Source: CAD feature listing. Evaluate the final solid. Frame: model axes, mm. Coordinates: 2 decimals unless noted, no trailing zeros. Write each loop counter-clockwise with the first axis right and the second up, starting at its lowest first coordinate (ties: lowest second). Pieces come first, ordered by that corner, then holes. Notation, with made-up numbers: M -7,-17 L -1,-17 A21 cw -1,20 Z; hole C 18.5,78.25 d6. An arc over 180 degrees is marked long. Write item = value, one per line. Start each with the question number.
1. Pin query (flat end, axial travel): pin 1 Ø5 at (x, y) = (0, 0) entering from -Z; pin 2 Ø2 at (x, z) = (3.5, 2) entering from -Y; pin 3 Ø1 at (x, z) = (-1, 3) entering from +Y; pin 4 Ø2 at (y, z) = (-3, 6.5) entering from -X. Return the tip coordinate at first contact, or that it passes through.
2. Section query A-A (y = 0). Output: boundary loops of the cut face in (x, z) (3 decimals), then the cut area to 3 significant figures.
3. Line query: line 1 along Y through (x, z) = (0, 6.25) (3 decimals); line 2 along Z through (x, y) = (0, 5); line 3 along Y through (x, z) = (0, 4.5) (3 decimals). Output: solid intervals per line, ascending.
4. Section query D-D (y = 7.75). Output: boundary loops of the cut face in (x, z).
5. Pull-direction query (Y, two-part tool) for faces 1 (the face through (0.34, -9.22, 3.88)), 2 (the face through (0.41, -3.15, 3.99)), 3 (the face through (-2.75, -12.4, 3.88)), 4 (the face through (0.662, 7.613, 2.297)); classes: pulls with the +Y half, pulls with the -Y half, needs draft (parallel to the pull), parting line crosses it, or undercut.
6. Section query B-B (x = 0). Output: boundary loops of the cut face in (y, z) (3 decimals).
```python
from build123d import *

# Parameters (mm, degrees)
SKETCH1_R                  = 12.7
BOSS_EXTRUDE1_DEPTH        = 7.874
F_1_4_0_2500_DOWEL_HOLE1_D = 6.35
F_1_8_0_1250_DOWEL_HOLE1_D = 3.175


with BuildPart() as part:
    # Sketch1 → Boss-Extrude1 (new body)
    with BuildSketch(Plane.XY):
        Circle(SKETCH1_R)
    extrude(amount=BOSS_EXTRUDE1_DEPTH)

    # 1/4 (0.2500) Dowel Hole1 (through all)
    with Locations(Plane(origin=(0, 0, 0), x_dir=(1, 0, 0), z_dir=(0, 0, -1))):
        with Locations((0, 0)):
            Hole(F_1_4_0_2500_DOWEL_HOLE1_D / 2)

    # 1/8 (0.1250) Dowel Hole1 (through all)
    with Locations(Plane.XY.offset(7.874)):
        with Locations((0, -7.669668031)):
            Hole(F_1_8_0_1250_DOWEL_HOLE1_D / 2)

    # Sketch7 → #8-32 Tapped Hole1 (revolve, cut)
    with BuildSketch(Plane(origin=(0, 0, 3.892930906), x_dir=(0, 0, -1), z_dir=(1, 0, 0))):
        Polygon((0, 0), (0, 13.97), (1.7272, 12.932193539), (1.7272, 0), align=None)
    revolve(axis=Axis((0, -6.35, 3.892930906), (0, 1, 0)), mode=Mode.SUBTRACT)


solid = part.part
```
Results are:
q1.pin_1 = through
q1.pin_2 = -12.45
q1.pin_3 = 12.66
q1.pin_4 = -12.54
q2.outline = M -12.7,0 L -3.175,0 L -3.175,7.874 L -12.7,7.874 Z; M 3.175,0 L 12.7,0 L 12.7,7.874 L 3.175,7.874 Z
q2.area = 150 mm^2
q3.line_1 = -12.7 to -9.257, -6.082 to -3.175, 3.175 to 12.7
q3.line_2 = 0 to 2.17, 5.62 to 7.87
q3.line_3 = -12.7 to -9.257, -6.082 to -3.175
q4.outline = M -10.06,0 L 10.06,0 L 10.06,7.87 L -10.06,7.87 Z; hole C 0,3.89 d3.45
q5.face_1 = undercut
q5.face_2 = undercut
q5.face_3 = parting line crosses it
q5.face_4 = needs draft
q6.outline = M -12.7,0 L -9.257,0 L -9.257,7.874 L -12.7,7.874 Z; M -6.082,0 L -3.175,0 L -3.175,7.874 L -6.082,7.874 Z; M 3.175,0 L 12.7,0 L 12.7,2.166 L 3.175,2.166 Z; M 3.175,5.62 L 12.7,5.62 L 12.7,7.874 L 3.175,7.874 Z
